Input: part model. Units: mm. Frame: model coordinates. A direction names the side the tool comes from. Coordinates: 2 decimals unless noted, no trailing zeros. Order: outer loops, then holes, each group sorted by start corner. A loop starts at its lowest first (then second) coordinate and runs counter-clockwise, first axis right, second up. Notation, with made-up numbers: M -33,29 L -26,29 A30 ccw -26,58 Z; hole C 7.25,-14 d6. An arc over 180 degrees is marked long. Answer in a Markdown table with one row per item.
from build123d import *

# Parameters (mm, degrees)
F1_DEPTH = 101.6
F3_DEPTH = 50.8
F4_R     = 25.4
F5_DEPTH = 88.9


with BuildPart() as f1:
    # F0 (on Front) → F1 (new body, symmetric)
    with BuildSketch(Plane.XZ):
        Polygon((0, 50.8), (0, 0), (254, 0), (254, 50.8), (127, 177.8), (76.2, 127), (152.4, 50.8), align=None)
    extrude(amount=F1_DEPTH, both=True)

    # F2 (on face) → F3 (cut)
    with BuildSketch(Plane.XY.offset(50.8)):
        Polygon((0, 101.6), (0, 50.8), (50.8, 101.6), align=None)
        Polygon((50.8, -101.6), (0, -50.8), (0, -101.6), align=None)
    extrude(amount=-F3_DEPTH, mode=Mode.SUBTRACT)

    # F4 (on face) → F5 (cut)
    with BuildSketch(Plane(origin=(152.4, 0, 152.4), x_dir=(0.707107, 0, -0.707107), z_dir=(0.707107, 0, 0.707107))):
        with Locations((2.178976, 0)):
            Circle(F4_R)
    extrude(amount=-F5_DEPTH, mode=Mode.SUBTRACT)


solid = f1.part
1) Material intervals for probe 1 along Z at (x, y) = (118.5, -16); probe 2 along Z at (x, y) = (31, -59); probe 3 along Z at (x, y) = (117.5, -11), sorted ascending.
Resolved:
| item | result |
|---|---|
| probe 1 | z = 0 to 50.8, 84.7 to 87.52, 143.32 to 169.3 |
| probe 2 | z = 0 to 50.8 |
| probe 3 | z = 0 to 50.8, 146.8 to 168.3 |
2) Mould query, pull axis Z, two halves, no side actions, for faces 1 (the face through (191.4, -1.4, 113.4)), 2 (the face through (146.027, 7.629, 108.684)), 3 (the face through (0, -1, 26)). Classes: +Z half, -Z half, draft (parallel to the pull), parting line (faces both ways), or undercut.
Resolved:
| item | result |
|---|---|
| face 1 | +Z half |
| face 2 | undercut |
| face 3 | draft |
3) Cut plane A-A, the plane y = 77. Output: boundary loops of the cut face in (x, z), and give its area (3 significant figures).
Resolved:
| item | result |
|---|---|
| outline | M 26.2,0 L 254,0 L 254,50.8 L 127,177.8 L 76.2,127 L 152.4,50.8 L 26.2,50.8 Z |
| area | 21,900 mm2 |
4) Cut plane C-C, the plane z = 30. Output: boundary loops of the cut face in (x, y), and give its area (3 significant figures).
Resolved:
| item | result |
|---|---|
| outline | M 0,-50.8 L 50.8,-101.6 L 254,-101.6 L 254,101.6 L 50.8,101.6 L 0,50.8 Z |
| area | 49,000 mm2 |
5) Contact query for flat-ended pins moving along their axis: pin 1 (2 mm diameter, centred on y = 31.5, z = 64.5, fed in from -X); pin 2 (12 mm diameter, centred on x = 78, z = 59.5, fed in from +Y). Output: stop coordinate, or through.
Resolved:
| item | result |
|---|---|
| pin 1 | stops at x = 137.7 |
| pin 2 | passes through |
6) Cut plane D-D, the plane x = 63. Output: boundary loops of the cut face in (y, z).
Resolved:
| item | result |
|---|---|
| outline | M -101.6,0 L 101.6,0 L 101.6,50.8 L -101.6,50.8 Z |
7) Cut plane B-B, the plane y = -12.5. Output: boundary loops of the cut face in (x, z), and give its area (3 significant figures).
Resolved:
| item | result |
|---|---|
| outline | M 0,0 L 254,0 L 254,50.8 L 169.58,135.22 L 118.78,84.42 L 152.4,50.8 L 0,50.8 Z; M 76.2,127 L 87.51,115.69 L 138.31,166.49 L 127,177.8 Z |
| area | 20,000 mm2 |
8) Reachability of faces 4 (the face through (102, -1.4, 152.8)), 5 (the face through (77, -1, 50.8)) from +Z, -Z, +X, -X, +Y, -Y: full face, straight path, thin tool, end or side. Return the list, or none.
Resolved:
| item | result |
|---|---|
| face 4 | +Z, -X, +Y, -Y |
| face 5 | -X, +Y, -Y |
